```python
from build123d import *

# Parameters (mm, degrees)
EXTRUDE_2_DEPTH     = 2
SKETCH_3_R          = 1.5
CUT_EXTRUDE_1_DEPTH = 95.361008897
EXTRUDE_3_DEPTH     = 1
DRAFT_4_ANGLE       = 43
SKETCH_6_W          = 6
SKETCH_6_H          = 10
EXTRUDE_4_DEPTH     = 5
SKETCH_7_W          = 6
SKETCH_7_H          = 10
EXTRUDE_5_DEPTH     = 5
CUT_EXTRUDE_2_DEPTH = 107.596038813
CUT_EXTRUDE_4_DEPTH = 107.596038813


with BuildPart() as part:
    # 草图1 → 凸台-拉伸2 (new body)
    with BuildSketch(Plane.XY):
        Polygon((0, 0), (0, 50), (20, 50), (20, 40), (60, 40), (60, 50), (80, 50), (80, 0), (60, 0), (60, 10), (20, 10), (20, 0), align=None)
    extrude(amount=EXTRUDE_2_DEPTH)

    # 草图3 → 切除-拉伸1 (cut, through all)
    with BuildSketch(Plane.XY.offset(2)):
        with Locations((10, 45)):
            Circle(SKETCH_3_R)
        with Locations((10, 5)):
            Circle(SKETCH_3_R)
        with Locations((70, 45)):
            Circle(SKETCH_3_R)
        with Locations((70, 5)):
            Circle(SKETCH_3_R)
    extrude(amount=-CUT_EXTRUDE_1_DEPTH, mode=Mode.SUBTRACT)

    # 草图5 → 凸台-拉伸3 (add)
    with BuildSketch(Plane.XY.offset(2)):
        with BuildLine():
            Line((0, 50), (6, 50))
            Line((6, 50), (6, 45))
            ThreePointArc((6, 45), (10, 41), (14, 45))
            Line((14, 45), (14, 50))
            Line((14, 50), (20, 50))
            Line((20, 50), (20, 40))
            Line((20, 40), (60, 40))
            Line((60, 40), (60, 50))
            Line((60, 50), (66, 50))
            Line((66, 50), (66, 45))
            ThreePointArc((66, 45), (70, 41), (74, 45))
            Line((74, 45), (74, 50))
            Line((74, 50), (80, 50))
            Line((80, 50), (80, 0))
            Line((80, 0), (74, 0))
            Line((74, 0), (74, 5))
            ThreePointArc((74, 5), (70, 9), (66, 5))
            Line((66, 5), (66, 0))
            Line((66, 0), (60, 0))
            Line((60, 0), (60, 10))
            Line((60, 10), (20, 10))
            Line((20, 10), (20, 0))
            Line((20, 0), (14, 0))
            Line((14, 0), (14, 5))
            ThreePointArc((14, 5), (10, 9), (6, 5))
            Line((6, 5), (6, 0))
            Line((6, 0), (0, 0))
            Line((0, 0), (0, 50))
        make_face()
    extrude(amount=EXTRUDE_3_DEPTH)

    # 拔模4
    draft_4_faces = [part.faces().sort_by_distance(p)[0] for p in [
        (40, 25, 3),
    ]]
    draft(draft_4_faces, Plane(origin=(20, 0, 2), x_dir=(-1, 0, 0), z_dir=(0, -1, 0)), DRAFT_4_ANGLE)

    # 草图6 → 凸台-拉伸4 (add)
    with BuildSketch(Plane(origin=(0, -1.496346075, 1.604634711), x_dir=(1, 0, 0), z_dir=(0, -0.6819983600624997, 0.7313537016191695))):
        with Locations((3, 7.04599508)):
            Rectangle(SKETCH_6_W, SKETCH_6_H)
    extrude(amount=EXTRUDE_4_DEPTH)

    # 草图7 → 凸台-拉伸5 (add)
    with BuildSketch(Plane(origin=(0, -1.496346075, 1.604634711), x_dir=(1, 0, 0), z_dir=(0, -0.6819983600624997, 0.7313537016191695))):
        with Locations((77, 7.04599508)):
            Rectangle(SKETCH_7_W, SKETCH_7_H)
    extrude(amount=EXTRUDE_5_DEPTH)

    # 草图8 → 切除-拉伸2 (cut, through all)
    with BuildSketch(Plane(origin=(80, 0, 0), x_dir=(0, 0, -1), z_dir=(1, 0, 0))):
        Polygon((-3, 0), (-9.836637305, 0), (-6.656768508, -3.4099918), align=None)
    extrude(amount=-CUT_EXTRUDE_2_DEPTH, mode=Mode.SUBTRACT)

    # 草图11 → 切除-拉伸4 (cut, through all)
    with BuildSketch(Plane(origin=(80, 0, 0), x_dir=(0, 0, -1), z_dir=(1, 0, 0))):
        Polygon((-3, 37), (-3, 13), (-11.020713736, 13), (-33.401075804, 37), align=None)
    extrude(amount=-CUT_EXTRUDE_4_DEPTH, mode=Mode.SUBTRACT)


solid = part.part
```
Check sheet for the modelled part. Datum: model origin and axes. Units: mm. A direction names the side the tool comes from. Round coordinates to 2 decimals unless told otherwise and drop trailing zeros. Write each loop counter-clockwise with the first axis right and the second up, starting at its lowest first coordinate (ties: lowest second). Pieces come first, ordered by that corner, then holes. Notation, with made-up numbers: (23.5, 46.5) -> (28.5, 46.5) arc R10 ccw to (28.5, 54.5) -> close; hole circle Ø3 at (41.25, -25.5). An arc over 180 degrees is marked (long way). Put each result on its own line as item: value.
(1) Mould release check, pull along Z, two halves, no side actions. Record for faces 4 (the face through (40.56, 25.35, 26.64)), 5 (the face through (41, 25, 3)), 6 (the face through (41, 37, 18)), 7 (the face through (20, 45, 24)): released by +Z, released by -Z, zero draft, split by the parting line, or undercut.
Values found:
face 4: released by +Z
face 5: undercut
face 6: undercut
face 7: zero draft
(2) Material ranges on line 1 (Y direction, x = 70, z = 0.8); line 2 (X direction, y = 48.5, z = 22.5); line 3 (Y direction, x = 7.5, z = 8), recorded low to high.
Values found:
line 1: y = 0 to 3.5, 6.5 to 43.5, 46.5 to 50
line 2: x = 0 to 6, 14 to 20, 60 to 66, 74 to 80
line 3: y = 8.12 to 13, 37 to 41.88
(3) Go/stop test with flat-tipped pins: pin 1 Ø4 at (x, y) = (9, 46) entering from +Z; pin 2 Ø9 at (x, z) = (36.5, 5.5) entering from +Y; pin 3 Ø9 at (x, y) = (70, 3) entering from +Z. Record where each tip stops, or that it passes through.
Values found:
pin 1: stops at z = 2
pin 2: stops at y = 40
pin 3: stops at z = 13.48
(4) Sectioned sample at A-A (z = 15.5). Enter the section's corners in (x, y).
Values found:
outline: (0, 13.4) -> (80, 13.4) -> (80, 17.8) -> (0, 17.8) -> close; (0, 37) -> (80, 37) -> (80, 50) -> (74, 50) -> (74, 45) arc R4 cw to (66, 45) -> (66, 50) -> (60, 50) -> (60, 40) -> (20, 40) -> (20, 50) -> (14, 50) -> (14, 45) arc R4 cw to (6, 45) -> (6, 50) -> (0, 50) -> close
(5) Sectioned sample at C-C (x = 70). Enter the section's corners in (y, z).
Values found:
outline: (0, 0) -> (3.5, 0) -> (3.5, 2) -> (0, 2) -> close; (6.5, 0) -> (43.5, 0) -> (43.5, 2) -> (41, 2) -> (41, 41.23) -> (9, 11.39) -> (9, 2) -> (6.5, 2) -> close; (46.5, 0) -> (50, 0) -> (50, 2) -> (46.5, 2) -> close; hole (13, 3) -> (37, 3) -> (37, 33.4) -> (13, 11.02) -> close
(6) Tool access check on faces 1 (the face through (40, 10, 6)), 2 (the face through (14, 3, 4)), 3 (the face through (60, 45, 24)). Record the directions out of +Z, -Z, +X, -X, +Y, -Y that give a thin tool (end or side, any length) a straight path to the whole face; none if there is none.
Values found:
face 1: +Z, -Z, -Y
face 2: +Z, -Y
face 3: +Z, -Z, +Y
(7) Sectioned sample at B-B (y = 33.5). Enter the section's corners in (x, z).
Values found:
outline: (0, 0) -> (80, 0) -> (80, 3) -> (0, 3) -> close; (0, 30.14) -> (80, 30.14) -> (80, 34.24) -> (0, 34.24) -> close
